Here's how the part is built. I have some questions about the finished solid (model axes, mm). Face numbers are marked on the shaded views. A direction names the side the tool comes from. Coordinates: 2 decimals unless noted, no trailing zeros. Write each loop counter-clockwise with the first axis right and the second up, starting at its lowest first coordinate (ties: lowest second). Pieces come first, ordered by that corner, then holes.
Item 1: Please list where these lines run through material, in increasing order: line 1 (X direction, y = 3.4, z = -6.75); line 2 (Z direction, x = 15.5, y = 4.6).
Item 2: For the marked faces 1, 2 and 3, which set-ups out of +Z, -Z, +X, -X, +Y, -Y let a thin tool reach every point of the face, with its end or its side?
Item 3: I want a section at B-B (x = 19). Please give me the cut outline in (y, z).
Item 4: I'm going to push flat-ended pins straight in: P1, Ø0.9, axis at y = 2, z = 8.5, coming from the +X side; P2, Ø2.5, axis at x = 2, y = 1.5, coming from the +Z side; P3, Ø2.5, axis at y = 1.5, z = 8.5, coming from the -X side; P4, Ø8, axis at x = -16, z = -7, coming from the -Y side. Where does each tip first touch, or does it pass through?
Item 5: I want a section at A-A (z = 8). Please give me the cut outline in (x, y).
Item 6: If we mould it in two halves opening along X, with no side actions, what happens to the marked faces 4, 5, 6 and 7? For each: pulls with the +X half, pulls with the -X half, needs draft (parallel to the pull), parting line crosses it, or undercut.
from build123d import *

# Parameters (mm, degrees)
SKETCH1_W           = 54
SKETCH1_H           = 13.1
SKETCH1_W_2         = 2.54
SKETCH1_H_2         = 3
BOSS_EXTRUDE1_DEPTH = 5


with BuildPart() as part:
    # Sketch1 → Boss-Extrude1 (new body)
    with BuildSketch(Plane(origin=(0, 0, 0), x_dir=(1, 0, 0), z_dir=(0, 1, 0))):
        Rectangle(SKETCH1_W, SKETCH1_H)
        with Locations((-16.962, -8.05)):
            Rectangle(SKETCH1_W_2, SKETCH1_H_2)
        with Locations((-5.654, -8.05)):
            Rectangle(SKETCH1_W_2, SKETCH1_H_2)
        with Locations((5.654, -8.05)):
            Rectangle(SKETCH1_W_2, SKETCH1_H_2)
        with Locations((16.962, -8.05)):
            Rectangle(SKETCH1_W_2, SKETCH1_H_2)
        with Locations((16.962, 8.05)):
            Rectangle(SKETCH1_W_2, SKETCH1_H_2)
        with Locations((5.654, 8.05)):
            Rectangle(SKETCH1_W_2, SKETCH1_H_2)
        with Locations((-5.654, 8.05)):
            Rectangle(SKETCH1_W_2, SKETCH1_H_2)
        with Locations((-16.962, 8.05)):
            Rectangle(SKETCH1_W_2, SKETCH1_H_2)
    extrude(amount=BOSS_EXTRUDE1_DEPTH)


solid = part.part
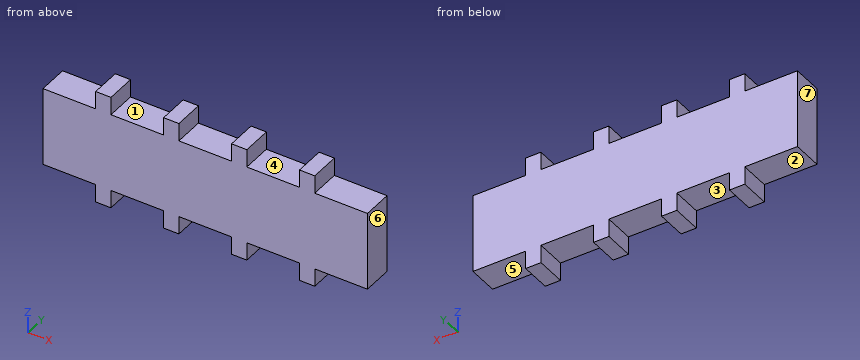
Answer:
1. line 1: x = -18.23 to -15.69, -6.92 to -4.38, 4.38 to 6.92, 15.69 to 18.23
1. line 2: z = -6.55 to 6.55
2. face 1: +Z, +Y, -Y
2. face 2: -Z, -X, +Y, -Y
2. face 3: -Z, +Y, -Y
3. outline: (0, -6.55) - (5, -6.55) - (5, 6.55) - (0, 6.55) - close
4. P1: stops at x = 18.23
4. P2: stops at z = 6.55
4. P3: stops at x = -18.23
4. P4: stops at y = 0
5. outline: (-18.23, 0) - (-15.69, 0) - (-15.69, 5) - (-18.23, 5) - close; (-6.92, 0) - (-4.38, 0) - (-4.38, 5) - (-6.92, 5) - close; (4.38, 0) - (6.92, 0) - (6.92, 5) - (4.38, 5) - close; (15.69, 0) - (18.23, 0) - (18.23, 5) - (15.69, 5) - close
6. face 4: undercut
6. face 5: needs draft
6. face 6: pulls with the +X half
6. face 7: pulls with the -X half
